```python
from build123d import *

# Parameters (mm, degrees)
F0_R     = 4.7625
F1_DEPTH = 38.1
F2_R     = 4.7625
F3_DEPTH = 24.385


with BuildPart() as f1:
    # F0 (on Top) → F1 (new body)
    with BuildSketch(Plane.XY):
        Polygon((0, 55.372), (0, 0), (37.338, 0), (37.338, 30.988), (74.676, 30.988), (74.676, 55.372), (37.338, 55.372), align=None)
        with Locations((19.05, 12.7)):
            Circle(F0_R, mode=Mode.SUBTRACT)
        with Locations((19.05, 42.672)):
            Circle(F0_R, mode=Mode.SUBTRACT)
    extrude(amount=F1_DEPTH)

    # F2 (on face) → F3 (cut, through all)
    with BuildSketch(Plane.XZ.offset(-30.988)):
        with Locations((61.976, 28.575)):
            Circle(F2_R)
        with Locations((61.341, 9.525)):
            Circle(F2_R)
    extrude(amount=-F3_DEPTH, mode=Mode.SUBTRACT)


solid = f1.part
```
Input: part model. Units: mm. Frame: model coordinates. A direction names the side the tool comes from. Coordinates: 2 decimals unless noted, no trailing zeros. Order: outer loops, then holes, each group sorted by start corner. A loop starts at its lowest first (then second) coordinate and runs counter-clockwise, first axis right, second up. Notation, with made-up numbers: (57.5, -23.75) - (87.5, -23.75) arc R32 ccw to (87.5, 6.25) - close; hole circle Ø2 at (-23.5, -31.5). An arc over 180 degrees is marked (long way). Return JSON: item names as keys, results as strings.
Q1. Draft query along Z for faces 3 (the flat face through (38, 55.372, 19)), 4 (the cylindrical face through (60.309, 43.009, 4.876)), 5 (the flat face through (29, 34, 0)), 6 (the cylindrical face through (64.17, 43.01, 24.35)). Return one class per face: +Z half, -Z half, draft (parallel to the pull), parting line (faces both ways), or undercut.
The answers:
{"face 3": "draft", "face 4": "undercut", "face 5": "-Z half", "face 6": "undercut"}
Q2. Cut plane A-A (z = 31.5). State how many separate pieces and enclosed holes the cut face has, then the cut area to 3 significant figures.
The answers:
{"separate pieces": "2", "enclosed holes": "2", "area": "2,650 mm2"}
Q3. Cut plane C-C (x = 19.05). Return loops of the section in (y, z), then the cut area to 3 significant figures.
The answers:
{"outline": "(0, 0) - (7.94, 0) - (7.94, 38.1) - (0, 38.1) - close; (17.46, 0) - (37.91, 0) - (37.91, 38.1) - (17.46, 38.1) - close; (47.43, 0) - (55.37, 0) - (55.37, 38.1) - (47.43, 38.1) - close", "area": "1,380 mm2"}
Q4. Access query for faces 1 (the cylindrical face through (14.292, 12.909, 18.783)), 2 (the flat face through (56, 30.988, 19)). Directions: +Z, -Z, +X, -X, +Y, -Y. A direction counts if a zero-diameter tool reaches every point of the face in a straight line with its end or side. Return the directions, or none.
The answers:
{"face 1": "+Z, -Z", "face 2": "+Z, -Z, +X, -Y"}
Q5. Cut plane D-D (y = 9). Return loops of the section in (x, z), then the cut area to 3 significant figures.
The answers:
{"outline": "(0, 0) - (16.05, 0) - (16.05, 38.1) - (0, 38.1) - close; (22.05, 0) - (37.34, 0) - (37.34, 38.1) - (22.05, 38.1) - close", "area": "1,190 mm2"}
Q6. Ray query, probe 1 along Y at (x, z) = (19, 9); probe 2 along X at (y, z) = (13, 20); probe 3 along Y at (x, z) = (18, 15.5). Return the intervals inside material, ascending.
The answers:
{"probe 1": "y = 0 to 7.94, 17.46 to 37.91, 47.43 to 55.37", "probe 2": "x = 0 to 14.3, 23.8 to 37.34", "probe 3": "y = 0 to 8.05, 17.35 to 38.03, 47.32 to 55.37"}
Q7. Cut plane B-B (y = 44). Return loops of the section in (x, z) (1 decimal), then the cut area to 3 significant figures.
The answers:
{"outline": "(0, 0) - (14.5, 0) - (14.5, 38.1) - (0, 38.1) - close; (23.6, 0) - (74.7, 0) - (74.7, 38.1) - (23.6, 38.1) - close; hole circle Ø9.5 at (61.3, 9.5); hole circle Ø9.5 at (62, 28.6)", "area": "2,350 mm2"}
Q8. First-contact query: pin 1 (6 mm diameter, centred on y = 27, z = 31.5, fed in from +X); pin 2 (7.5 mm diameter, centred on x = 19.05, y = 12.7, fed in from -Z). Flat tips, straight axial feed; report the tip coordinate or a pass-through.
The answers:
{"pin 1": "stops at x = 37.34", "pin 2": "passes through"}
